Geometry check sheet. Reference: the model listing, model coordinates, mm. Round coordinates to 2 decimals unless told otherwise and drop trailing zeros. Write each loop counter-clockwise with the first axis right and the second up, starting at its lowest first coordinate (ties: lowest second). Pieces come first, ordered by that corner, then holes. Notation, with made-up numbers: M 42.25,82 L 52.25,82 A11 ccw 52.25,98 Z; hole C -9,-38.5 d11. An arc over 180 degrees is marked long. Put each result on its own line as item: value. Start each with the question number.
(1) Material ranges on probe 1 along Y at (x, z) = (-20, -637) (3 decimals); probe 2 along Y at (x, z) = (0, -19.5), recorded low to high.
(2) Section check A-A on x = 0. Record the cut outline in (y, z) (1 decimal).
(3) Gauge pin test, flat ends, axial feed: pin 1 (1 mm diameter, centred on x = -13.5, y = 10, fed in from -Z); pin 2 (13.5 mm diameter, centred on x = 0.5, y = -2.5, fed in from -Z). Record the tip position at first contact, or that the pin passes through.
(4) Section check B-B on z = -652. Record the cut outline in (x, y) (3 decimals), then the cut area to 3 significant figures.
Autodesk Inventor part; units mm, degrees
ref_plane "YZ Plane" through (0, 0, 0) normal (1, 0, 0) x (0, 1, 0)
ref_plane "XZ Plane" through (0, 0, 0) normal (0, 1, 0) x (-1, 0, 0)
ref_plane "XY Plane" through (0, 0, 0) normal (0, 0, 1) x (1, 0, 0)
sketch "Sketch1" plane through (0, 0, 0) normal (0, 0, 1) x (1, 0, 0)
  line L0 (-25.4, -25.4) -> (25.4, -25.4)
  line L1 (25.4, -25.4) -> (25.4, 25.4)
  line L2 (25.4, 25.4) -> (-25.4, 25.4)
  line L3 (-25.4, 25.4) -> (-25.4, -25.4)
  line L4 (-25.4, -25.4) -> (25.4, 25.4) construction
  line L5 (25.4, -25.4) -> (-25.4, 25.4) construction
  line L6 (-22.225, -22.225) -> (22.225, -22.225)
  line L7 (22.225, -22.225) -> (22.225, 22.225)
  line L8 (22.225, 22.225) -> (-22.225, 22.225)
  line L9 (-22.225, 22.225) -> (-22.225, -22.225)
  line L10 (-22.225, -22.225) -> (22.225, 22.225) construction
  line L11 (22.225, -22.225) -> (-22.225, 22.225) construction
  point P0 (0, 0)
  dimension "d0" = 50.8
  dimension "d1" = 50.8
  dimension "d2" = 3.175
  dimension "d3" = 3.175
extrude "Extrusion1" add sketch "Sketch1" against normal blind 1447.8
sketch "Sketch2" plane through (0, 0, 0) normal (0, 0, 1) x (1, 0, 0)
  circle A0 centre (0, 0) radius 14.2875
  line L0 (-22.225, -22.225) -> (22.225, -22.225)
  line L1 (22.225, -22.225) -> (22.225, 22.225)
  line L2 (22.225, 22.225) -> (-22.225, 22.225)
  line L3 (-22.225, 22.225) -> (-22.225, -22.225)
  line L4 (-22.225, -22.225) -> (22.225, 22.225) construction
  line L5 (22.225, -22.225) -> (-22.225, 22.225) construction
  dimension "d6" = 28.575
extrude "Extrusion2" add sketch "Sketch2" against normal blind 25.4
properties part number "2x2x1_8_tubeForLift" material "Aluminum 6061"
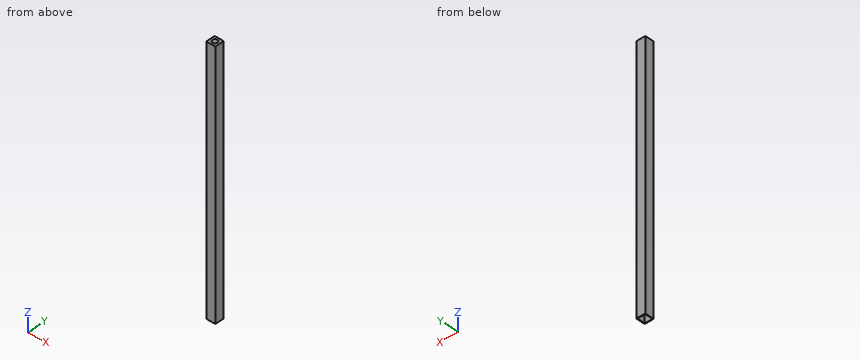
Answers follow:
1. probe 1: y = -25.4 to -22.225, 22.225 to 25.4
1. probe 2: y = -25.4 to -14.29, 14.29 to 25.4
2. outline: M -25.4,-1447.8 L -22.2,-1447.8 L -22.2,-25.4 L -14.3,-25.4 L -14.3,0 L -25.4,0 Z; M 14.3,-25.4 L 22.2,-25.4 L 22.2,-1447.8 L 25.4,-1447.8 L 25.4,0 L 14.3,0 Z
3. pin 1: stops at z = -25.4
3. pin 2: passes through
4. outline: M -25.4,-25.4 L 25.4,-25.4 L 25.4,25.4 L -25.4,25.4 Z; hole M -22.225,-22.225 L 22.225,-22.225 L 22.225,22.225 L -22.225,22.225 Z
4. area: 605 mm^2
